Verification items for the finished model (mm, model axes). Face numbers are marked on the shaded views. A direction names the side the tool comes from. Coordinates: 2 decimals unless noted, no trailing zeros. Loops run counter-clockwise (first coordinate to the right, second up) from the corner with the lowest first, then second, coordinate; pieces in that order, holes last. Notation, with made-up numbers: (45, 52.25) -> (95, 52.25) arc R24 ccw to (95, 88.25) -> close; hole circle Ø6 at (82, 8.25). An arc over 180 degrees is marked (long way). Answer as a JSON object with one key per item and string values. Group by question number.
Q1. Scan lines: L1, parallel to Y at x = -0.75, z = -3; L2, parallel to Z at x = 3, y = 0.4; L3, parallel to Z at x = -3, y = 0.1. Record each from-to range of solid material in increasing order.
Q2. Cross-section at B-B on x = 2.25. Record the boundary of the cut face in (y, z), and give its area (3 significant figures).
Q3. Cross-section at D-D on x = 0. Record the boundary of the cut face in (y, z).
Q4. Cross-section at A-A on z = 0. Record the boundary of the cut face in (x, y).
Q5. Set-up check for the marked faces 1 and 2: record each of +Z, -Z, +X, -X, +Y, -Y from which the full face is reachable in a straight line by a thin tool's end or side.
Q6. Gauge pin test, flat ends, axial feed: pin 1 Ø0.5 at (y, z) = (11, 0) entering from -X; pin 2 Ø6 at (x, y) = (-3.5, 3.5) entering from -Z; pin 3 Ø0.7 at (x, z) = (3, 0) entering from -Y; pin 4 Ø2 at (x, z) = (1.5, 1) entering from -Y. Record the tip position at first contact, or that the pin passes through.
Q7. Cross-section at C-C on y = 6. Record the boundary of the cut face in (x, z).
```python
from build123d import *

# Parameters (mm, degrees)
BOSS_EXTRUDE1_DEPTH = 11.5
SKETCH3_W           = 1
SKETCH3_H           = 1
CUT_EXTRUDE1_DEPTH  = 0.5
FILLET1_R           = 0.5
FILLET2_R           = 0.5
SKETCH4_R           = 2
BOSS_EXTRUDE3_DEPTH = 0.25
SKETCH5_R           = 0.25
BOSS_EXTRUDE4_DEPTH = 2.5
SKETCH6_R           = 0.376312749
SKETCH6_R_2         = 0.431953985
CUT_EXTRUDE2_DEPTH  = 0.5


with BuildPart() as part:
    # Sketch1 → Boss-Extrude1 (new body)
    with BuildSketch(Plane(origin=(0, 0, 0), x_dir=(1, 0, 0), z_dir=(0, 1, 0))):
        with BuildLine():
            Line((-3, 4), (3, 4))
            ThreePointArc((3, 4), (5, 0), (3, -4))
            Line((3, -4), (-3, -4))
            ThreePointArc((-3, -4), (-5, 0), (-3, 4))
        make_face()
    extrude(amount=BOSS_EXTRUDE1_DEPTH)

    # Sketch3 → Cut-Extrude1 (cut)
    with BuildSketch(Plane(origin=(5, 0, 0), x_dir=(0, 0, -1), z_dir=(1, 0, 0))):
        with Locations((0, 11)):
            Rectangle(SKETCH3_W, SKETCH3_H)
    cut_extrude1 = extrude(amount=-CUT_EXTRUDE1_DEPTH, mode=Mode.SUBTRACT)

    # Mirror1: Cut-Extrude1 across plane
    add(cut_extrude1.mirror(Plane(origin=(0, 0, 0), x_dir=(0, 0, 1), z_dir=(1, 0, 0))), mode=Mode.SUBTRACT)

    # Fillet1
    fillet1_edges = [part.edges().sort_by_distance(p)[0] for p in [
        (-3, 5.75, -4),
        (-3, 5.75, 4),
        (3, 5.75, 4),
        (3, 5.75, -4),
    ]]
    fillet(fillet1_edges, radius=FILLET1_R)

    # Fillet2
    fillet2_edges = [part.edges().sort_by_distance(p)[0] for p in [
        (-5, 0, 0),
        (0, 0, -4),
        (5, 0, 0),
        (0, 0, 4),
        (2.995093791, 0, 3.971404521),
        (-2.995093791, 0, 3.971404521),
        (2.995093791, 0, -3.971404521),
        (-2.995093791, 0, -3.971404521),
    ]]
    fillet(fillet2_edges, radius=FILLET2_R)

    # Sketch4 → Boss-Extrude3 (add)
    with BuildSketch(Plane.XZ):
        Circle(SKETCH4_R)
    extrude(amount=BOSS_EXTRUDE3_DEPTH)

    # Sketch5 → Boss-Extrude4 (add)
    with BuildSketch(Plane.XZ.offset(0.25)):
        Circle(SKETCH5_R)
    extrude(amount=BOSS_EXTRUDE4_DEPTH)

    # Sketch6 → Cut-Extrude2 (cut)
    with BuildSketch(Plane.XZ):
        with Locations((-3, 0)):
            Circle(SKETCH6_R)
        with Locations((3, 0)):
            Circle(SKETCH6_R_2)
    extrude(amount=-CUT_EXTRUDE2_DEPTH, mode=Mode.SUBTRACT)


solid = part.part
```
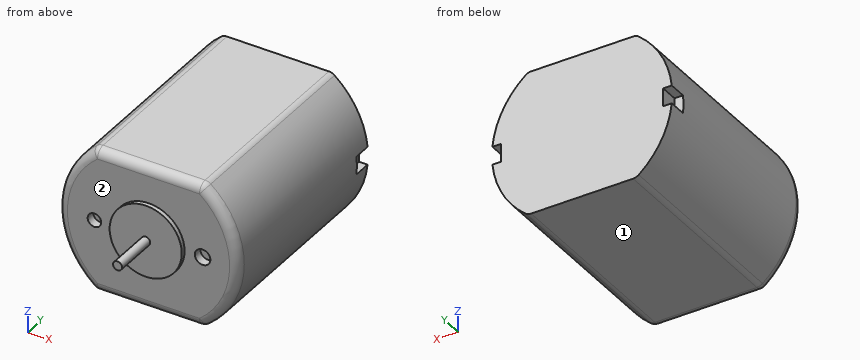
Computed values:
{
 "1": {"L1": "y = 0 to 11.5", "L2": "z = -3.96 to -0.43, 0.43 to 3.96", "L3": "z = -3.75 to -0.38, 0.38 to 3.75"},
 "2": {"outline": "(0, -3.5) arc R0.5 ccw to (0.5, -4) -> (11.5, -4) -> (11.5, 4) -> (0.5, 4) arc R0.5 ccw to (0, 3.5) -> close", "area": "91.9 mm²"},
 "3": {"outline": "(-2.75, -0.25) -> (-0.25, -0.25) -> (-0.25, -2) -> (0, -2) -> (0, -3.5) arc R0.5 ccw to (0.5, -4) -> (11.5, -4) -> (11.5, 4) -> (0.5, 4) arc R0.5 ccw to (0, 3.5) -> (0, 2) -> (-0.25, 2) -> (-0.25, 0.25) -> (-2.75, 0.25) -> close"},
 "4": {"outline": "(-5, 0.5) arc R0.5 ccw to (-4.5, 0) -> (-3.38, 0) -> (-3.38, 0.5) -> (-2.62, 0.5) -> (-2.62, 0) -> (-2, 0) -> (-2, -0.25) -> (-0.25, -0.25) -> (-0.25, -2.75) -> (0.25, -2.75) -> (0.25, -0.25) -> (2, -0.25) -> (2, 0) -> (2.57, 0) -> (2.57, 0.5) -> (3.43, 0.5) -> (3.43, 0) -> (4.5, 0) arc R0.5 ccw to (5, 0.5) -> (5, 10.5) -> (4.5, 10.5) -> (4.5, 11.5) -> (-4.5, 11.5) -> (-4.5, 10.5) -> (-5, 10.5) -> close"},
 "5": {"face 1": "-Z, +X, -X, +Y, -Y", "face 2": "-Y"},
 "6": {"pin 1": "stops at x = -4.5", "pin 2": "stops at z = -4", "pin 3": "stops at y = 0.5", "pin 4": "stops at y = -0.25"},
 "7": {"outline": "(-3.14, -3.89) arc R0.5 ccw to (-2.83, -4) -> (2.83, -4) arc R0.5 ccw to (3.14, -3.89) arc R5 ccw to (3.14, 3.89) arc R0.5 ccw to (2.83, 4) -> (-2.83, 4) arc R0.5 ccw to (-3.14, 3.89) arc R5 ccw to start"}
}
